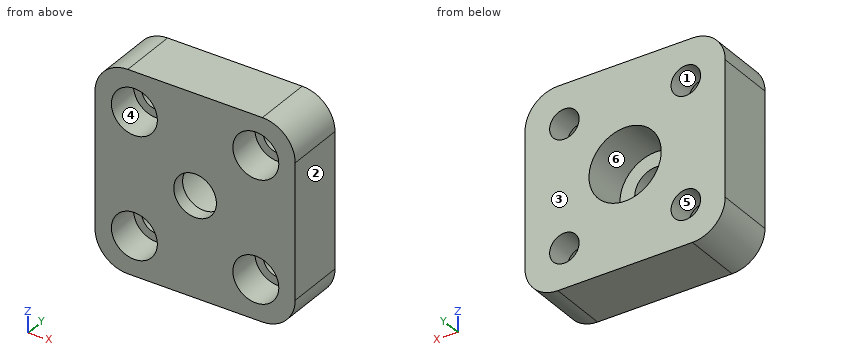
Autodesk Inventor part; units mm, degrees
ref_plane "YZ Plane" through (0, 0, 0) normal (1, 0, 0) x (0, 1, 0)
ref_plane "XZ Plane" through (0, 0, 0) normal (0, 1, 0) x (-1, 0, 0)
ref_plane "XY Plane" through (0, 0, 0) normal (0, 0, 1) x (1, 0, 0)
sketch "Sketch1" plane through (0, 0, 0) normal (0, 1, 0) x (-1, 0, 0)
  line L0 (-15.25, -15.25) -> (15.25, -15.25)
  line L1 (15.25, -15.25) -> (15.25, 15.25)
  line L2 (15.25, 15.25) -> (-15.25, 15.25)
  line L3 (-15.25, 15.25) -> (-15.25, -15.25)
  line L4 (-15.25, -15.25) -> (15.25, 15.25) construction
  line L5 (15.25, -15.25) -> (-15.25, 15.25) construction
  point P0 (0, 0)
  dimension "d0" = 30.5
  dimension "d1" = 30.5
extrude "Extrusion1" add sketch "Sketch1" along normal blind 9
hole "Hole5" at (0, 9, 0) direction (0, -1, 0) diameter 6.5 end through all counterbore diameter 11 counterbore depth 7
fillet "Fillet1" radius 5 1 edges at (15.25, 4.5, 15.25)
fillet "Fillet2" radius 5 1 edges at (15.25, 4.5, -15.25)
fillet "Fillet3" radius 5 1 edges at (-15.25, 4.5, -15.25)
fillet "Fillet4" radius 5 1 edges at (-15.25, 4.5, 15.25)
hole "Hole10" at (-9.25, 0, -9.25) direction (0, 1, 0) diameter 4.5 end through all counterbore diameter 7 counterbore depth 5
hole "Hole11" at (-9.25, 0, 9.25) direction (0, 1, 0) diameter 4.5 end through all counterbore diameter 7 counterbore depth 5
hole "Hole12" at (9.25, 0, 9.25) direction (0, 1, 0) diameter 4.5 end through all counterbore diameter 7 counterbore depth 5
hole "Hole13" at (9.25, 0, -9.25) direction (0, 1, 0) diameter 4.5 end through all counterbore diameter 7 counterbore depth 5
properties part number "OdourPort_minimal_backplate"
Design review of the part built by this model. Coordinates are the model's own, in mm. Face numbers are marked on the shaded views. A direction names the side the tool comes from. Coordinates: 2 decimals unless noted, no trailing zeros. Write each loop counter-clockwise with the first axis right and the second up, starting at its lowest first coordinate (ties: lowest second). Pieces come first, ordered by that corner, then holes. Notation, with made-up numbers: (48, -3) -> (91, -3) arc R5 ccw to (91, 5) -> close; hole circle Ø7 at (-11, -36.75). An arc over 180 degrees is marked (long way). Write each question's results on one line, items separated by ' | '. Start each with the question number.
(1) Take a section at B-B on y = 2.5. Write out the cut boundary in (x, z).
(2) The part is to be moulded in two halves that separate along X. For the marked faces 1, 2 and 3, say which applies: pulls with the +X half, pulls with the -X half, needs draft (parallel to the pull), parting line crosses it, or undercut.
(3) For line 1 along X through (y, z) = (6.2, -9.25); line 2 along Z through (x, y) = (-9.25, 2.45), list the stretches that pass through material, from the lowest coordinate up. Write a range as from..to.
(4) Tool access review of the marked faces 4, 5 and 6: name each direction out of +Z, -Z, +X, -X, +Y, -Y from which nothing blocks a thin tool from reaching the whole face with its end or side.
(5) Clearance check with flat-ended pins moving along their axes: P1, Ø10, axis at x = 0, z = 0, coming from the +Y side; P2, Ø6, axis at x = 9.25, z = -9.25, coming from the -Y side. State where each tip first meets the part, or that it passes through.
(6) Take a section at D-D on x = 0. Write out the cut boundary in (y, z), and give its area (4 significant figures).
(7) Take a section at A-A on x = -9.25. Write out the cut boundary in (y, z).
(8) Take a section at C-C on z = 0. Write out the cut boundary in (x, y).
Results found:
1) outline: (-15.25, -10.25) arc R5 ccw to (-10.25, -15.25) -> (10.25, -15.25) arc R5 ccw to (15.25, -10.25) -> (15.25, 10.25) arc R5 ccw to (10.25, 15.25) -> (-10.25, 15.25) arc R5 ccw to (-15.25, 10.25) -> close; hole circle Ø7 at (-9.25, -9.25); hole circle Ø7 at (-9.25, 9.25); hole circle Ø11 at (0, 0); hole circle Ø7 at (9.25, -9.25); hole circle Ø7 at (9.25, 9.25)
2) face 1: undercut | face 2: pulls with the +X half | face 3: needs draft
3) line 1: x = -15.25..-11.5, -7..7, 11.5..15.25 | line 2: z = -15.25..-12.75, -5.75..5.75, 12.75..15.25
4) face 4: -Y | face 5: +Y, -Y | face 6: +Y
5) P1: stops at y = 2 | P2: stops at y = 5
6) outline: (0, -15.25) -> (9, -15.25) -> (9, -5.5) -> (2, -5.5) -> (2, -3.25) -> (0, -3.25) -> close; (0, 3.25) -> (2, 3.25) -> (2, 5.5) -> (9, 5.5) -> (9, 15.25) -> (0, 15.25) -> close | area: 184.5 mm2
7) outline: (0, -15.25) -> (9, -15.25) -> (9, -11.5) -> (5, -11.5) -> (5, -12.75) -> (0, -12.75) -> close; (0, -5.75) -> (5, -5.75) -> (5, -7) -> (9, -7) -> (9, 7) -> (5, 7) -> (5, 5.75) -> (0, 5.75) -> close; (0, 12.75) -> (5, 12.75) -> (5, 11.5) -> (9, 11.5) -> (9, 15.25) -> (0, 15.25) -> close
8) outline: (-15.25, 0) -> (-3.25, 0) -> (-3.25, 2) -> (-5.5, 2) -> (-5.5, 9) -> (-15.25, 9) -> close; (3.25, 0) -> (15.25, 0) -> (15.25, 9) -> (5.5, 9) -> (5.5, 2) -> (3.25, 2) -> close
